Can you work these out from the model? Positions are in its coordinate system, mm. A direction names the side the tool comes from. Round coordinates to 2 decimals unless told otherwise and drop trailing zeros. Loops run counter-clockwise (first coordinate to the right, second up) from the corner with the lowest first, then second, coordinate; pieces in that order, holes last. Notation, with made-up numbers: M 25.25,64 L 47.25,64 A16 ccw 47.25,69 Z; hole C 84.25,8.5 d6. An arc over 180 degrees is marked long. Return JSON: item names as keys, results as strings.
```python
from build123d import *

# Parameters (mm, degrees)
SKETCH_1_W           = 10
SKETCH_1_H           = 15.42
SKETCH_1_H_2         = 10
SKETCH_1_W_2         = 31
SKETCH_1_H_3         = 20.133
EXTRUDE_1_DEPTH      = 1
EXTRUDE_2_DEPTH      = 4
EXTRUDE_2_DEPTH_BACK = 1
SKETCH_3_W           = 10
SKETCH_3_H           = 40.84
SKETCH_3_H_2         = 50.266
EXTRUDE_3_DEPTH      = 2


with BuildPart() as part:
    # Sketch 1 → Extrude 1 (new body)
    with BuildSketch(Plane(origin=(0, 0, 0), x_dir=(1, 0, 0), z_dir=(0, 1, 0))):
        with Locations((-20.5, 12.71)):
            Rectangle(SKETCH_1_W, SKETCH_1_H)
        with Locations((-20.5, 0)):
            Rectangle(SKETCH_1_W, SKETCH_1_H_2)
        with Locations((-20.5, -12.71)):
            Rectangle(SKETCH_1_W, SKETCH_1_H)
        Rectangle(SKETCH_1_W_2, SKETCH_1_H_2)
        with Locations((20.5, 15.0665)):
            Rectangle(SKETCH_1_W, SKETCH_1_H_3)
        with Locations((20.5, 0)):
            Rectangle(SKETCH_1_W, SKETCH_1_H_2)
        with Locations((20.5, -15.0665)):
            Rectangle(SKETCH_1_W, SKETCH_1_H_3)
    extrude(amount=EXTRUDE_1_DEPTH)



with BuildPart() as body_2:
    # Sketch 2 → Extrude 2 (new body, two sides)
    with BuildSketch(Plane(origin=(0, 1, 0), x_dir=(1, 0, 0), z_dir=(0, 1, 0))) as extrude_2_sk:
        Polygon((-26.5, 21.42), (-26.5, -21.42), (-14.5, -21.42), (-14.5, -6), (14.5, -6), (14.5, -26.133), (26.5, -26.133), (26.5, 26.133), (14.5, 26.133), (14.5, 6), (-14.5, 6), (-14.5, 21.42), align=None)
        Polygon((-15.5, -5), (15.5, -5), (15.5, -25.133), (25.5, -25.133), (25.5, 25.133), (15.5, 25.133), (15.5, 5), (-15.5, 5), (-15.5, 20.42), (-25.5, 20.42), (-25.5, -20.42), (-15.5, -20.42), align=None, mode=Mode.SUBTRACT)
    extrude(amount=EXTRUDE_2_DEPTH)
    extrude(extrude_2_sk.sketch, amount=-EXTRUDE_2_DEPTH_BACK)


with BuildPart() as part_1:
    add(part.part)

    add(body_2.part)  # Extrude 3 merges body 2
    # Sketch 3 → Extrude 3 (add)
    with BuildSketch(Plane(origin=(0, 1, 0), x_dir=(1, 0, 0), z_dir=(0, 1, 0))):
        with Locations((-20.5, 0)):
            Rectangle(SKETCH_3_W, SKETCH_3_H)
        with Locations((20.5, 0)):
            Rectangle(SKETCH_3_W, SKETCH_3_H_2)
    extrude(amount=EXTRUDE_3_DEPTH)


solid = part_1.part
```
Q1. Thinking about a two-plate mould opening in Z: for faces 6 (the flat face through (0, 3, 5)), 7 (the flat face through (-26.5, 3, 0)), 8 (the flat face through (20, 3, 26.133)), which applies, pulls with the +Z half, pulls with the -Z half, needs draft (parallel to the pull), parting line crosses it, or undercut?
Results:
{"face 6": "undercut", "face 7": "needs draft", "face 8": "pulls with the +Z half"}
Q2. Suppose I cut it at A-A, the plane y = 3.95. Please give me the cut outline in (x, z).
Results:
{"outline": "M -26.5,-21.42 L -14.5,-21.42 L -14.5,-6 L 14.5,-6 L 14.5,-26.13 L 26.5,-26.13 L 26.5,26.13 L 14.5,26.13 L 14.5,6 L -14.5,6 L -14.5,21.42 L -26.5,21.42 Z; hole M -25.5,-20.42 L -15.5,-20.42 L -15.5,-5 L 15.5,-5 L 15.5,-25.13 L 25.5,-25.13 L 25.5,25.13 L 15.5,25.13 L 15.5,5 L -15.5,5 L -15.5,20.42 L -25.5,20.42 Z"}
Q3. Suppose I cut it at C-C, the plane x = 19.5. Please give me the cut outline in (y, z), plus the area to 3 significant figures.
Results:
{"outline": "M 0,-26.13 L 5,-26.13 L 5,-25.13 L 3,-25.13 L 3,25.13 L 5,25.13 L 5,26.13 L 0,26.13 Z", "area": "161 mm2"}
Q4. If I drill on line 1 along X through (y, z) = (4.1, -11.5); line 2 along Z through (x, y) = (2.5, 2.05); line 3 along Z through (x, y) = (20.5, 4.55), over which ranges is the centre line in solid material (lowest first)?
Results:
{"line 1": "x = -26.5 to -25.5, -15.5 to -14.5, 14.5 to 15.5, 25.5 to 26.5", "line 2": "z = -6 to -5, 5 to 6", "line 3": "z = -26.13 to -25.13, 25.13 to 26.13"}
Q5. I'm going to push flat-ended pins straight in: pin 1 Ø2 at (x, y) = (-0.5, 3) entering from -Z; pin 2 Ø2 at (x, y) = (-19, 4) entering from -Z; pin 3 Ø2 at (x, z) = (12.5, 2) entering from +Y. Where does each tip first touch, or does it pass through?
Results:
{"pin 1": "stops at z = -6", "pin 2": "stops at z = -21.42", "pin 3": "stops at y = 1"}
Q6. Suppose I cut it at D-D, the plane z = -0.5. Please give me the cut outline in (x, y).
Results:
{"outline": "M -26.5,0 L 26.5,0 L 26.5,5 L 25.5,5 L 25.5,3 L 15.5,3 L 15.5,1 L -15.5,1 L -15.5,3 L -25.5,3 L -25.5,5 L -26.5,5 Z"}
Q7. On a 3-axis mill with a long thin cutter (end or side, diameter ignored), from which of +Z, -Z, +X, -X, +Y, -Y can I reach the whole of each face in a straight line? I mean faces 1 (the flat face through (-14.5, 3, 14)), 2 (the flat face through (-25.5, 4, 0)), 3 (the flat face through (-20, 3, -21.42)), 4 (the flat face through (26.5, 3, 0)), 5 (the flat face through (-21, 3, 21.42)). Say none if no direction works.
Results:
{"face 1": "+Z, +Y, -Y", "face 2": "+Y", "face 3": "-Z, -X, +Y, -Y", "face 4": "+Z, -Z, +X, +Y, -Y", "face 5": "+Z, -X, +Y, -Y"}
Q8. Suppose I cut it at B-B, the plane z = -7. Please give me the cut outline in (x, y), plus the area to 3 significant figures.
Results:
{"outline": "M -26.5,0 L -14.5,0 L -14.5,5 L -15.5,5 L -15.5,3 L -25.5,3 L -25.5,5 L -26.5,5 Z; M 14.5,0 L 26.5,0 L 26.5,5 L 25.5,5 L 25.5,3 L 15.5,3 L 15.5,5 L 14.5,5 Z", "area": "80.0 mm2"}
